Job drawing, mm, ordinate dimensions from the low corner. One solid piece. A direction names the side the tool comes from. Round coordinates to 2 decimals unless told otherwise and drop trailing zeros. Write each loop counter-clockwise with the first axis right and the second up, starting at its lowest first coordinate (ties: lowest second). Pieces come first, ordered by that corner, then holes. Notation, with made-up numbers: M 12.5,-4 L 36.5,-4 A23 cw 36.5,34 Z; hole C 34.5,49 d1. An arc over 180 degrees is marked long. Answer as a JSON object with one key per item and string values. Group by question number.
1. Drop a flat-ended pin along its axis: pin 1 (4 mm diameter, centred on x = 6.5, y = 6.5, fed in from +Z). Give the stop position or say it passes through.
2. Two-plate mould, pull along X, no slides. Class the marked faces 3, 4 and 5: +X half, -X half, draft (parallel to the pull), parting line (faces both ways), or undercut.
3. Band-saw the part on B-B, the plane y = 9.5. Write the cut outline in (x, z).
4. Band-saw the part on C-C, the plane z = 6.5. Write the cut outline in (x, y).
5. Which spindle directions (+Z, -Z, +X, -X, +Y, -Y) get a long thin tool onto all of the face, cutting with end or side? Do the marked faces 1 and 2. Say none if no direction does.
6. Drill centre lines: line 1 (Y direction, x = 23, z = 19.5); line 2 (X direction, y = 10.5, z = 12.25); line 3 (Y direction, x = 15.75, z = 1.45). Where is each one in solid material? Low to high. Write a range as from..to.
7. Band-saw the part on D-D, the plane y = 15.75. Write the cut outline in (x, z).
8. Band-saw the part on A-A, the plane x = 15.75. Write the cut outline in (y, z).
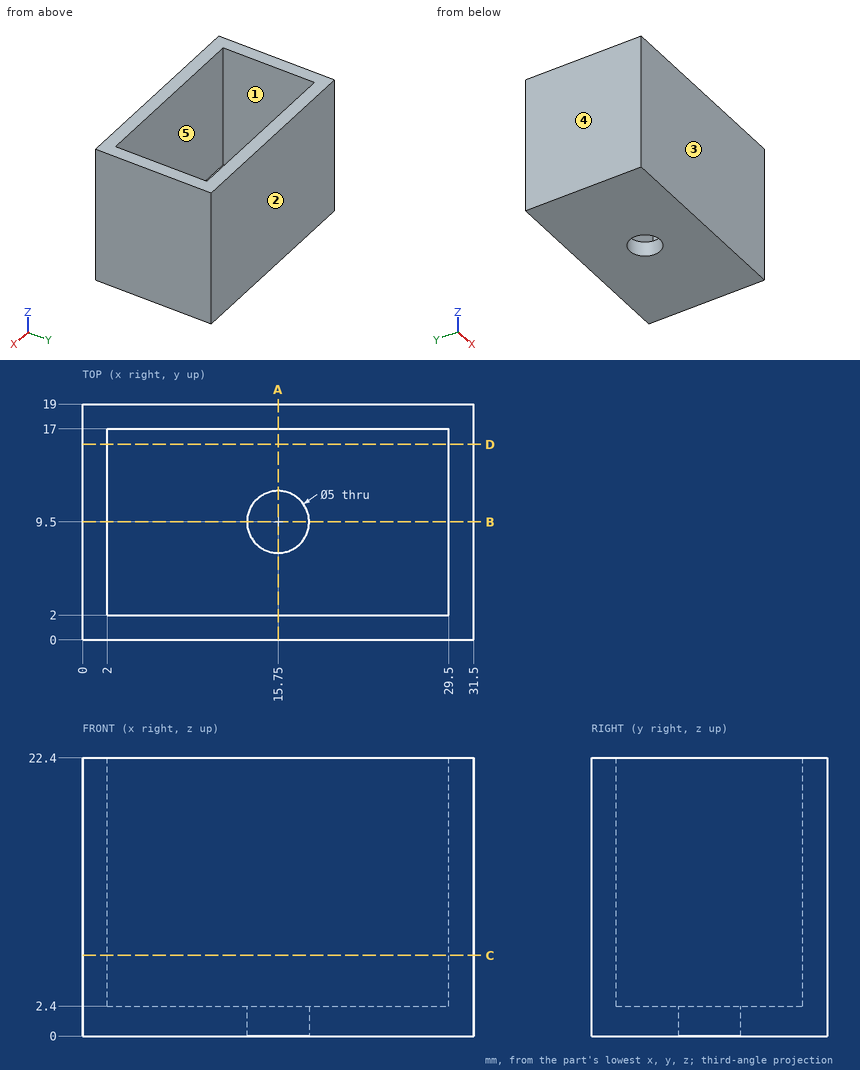
Worked answers:
{
 "1": {"pin 1": "stops at z = 2.4"},
 "2": {"face 3": "draft", "face 4": "-X half", "face 5": "undercut"},
 "3": {"outline": "M 0,0 L 13.25,0 L 13.25,2.4 L 2,2.4 L 2,22.4 L 0,22.4 Z; M 18.25,0 L 31.5,0 L 31.5,22.4 L 29.5,22.4 L 29.5,2.4 L 18.25,2.4 Z"},
 "4": {"outline": "M 0,0 L 31.5,0 L 31.5,19 L 0,19 Z; hole M 2,2 L 29.5,2 L 29.5,17 L 2,17 Z"},
 "5": {"face 1": "+Z", "face 2": "+Z, -Z, +X, -X, +Y"},
 "6": {"line 1": "y = 0..2, 17..19", "line 2": "x = 0..2, 29.5..31.5", "line 3": "y = 0..7, 12..19"},
 "7": {"outline": "M 0,0 L 31.5,0 L 31.5,22.4 L 29.5,22.4 L 29.5,2.4 L 2,2.4 L 2,22.4 L 0,22.4 Z"},
 "8": {"outline": "M 0,0 L 7,0 L 7,2.4 L 2,2.4 L 2,22.4 L 0,22.4 Z; M 12,0 L 19,0 L 19,22.4 L 17,22.4 L 17,2.4 L 12,2.4 Z"}
}
